```python
from build123d import *

# Parameters (mm, degrees)
F0_W     = 50
F0_H     = 80
F1_DEPTH = 60
F3_DEPTH = 80.001
F6_DEPTH = 66.156149
F7_W     = 5
F7_H     = 12.45938
F8_DEPTH = 43.57978


with BuildPart() as f1:
    # F0 (on Top) → F1 (new body)
    with BuildSketch(Plane.XY):
        with Locations((25, 40)):
            Rectangle(F0_W, F0_H)
    extrude(amount=F1_DEPTH)

    # F2 (on face) → F3 (cut, through all)
    with BuildSketch(Plane.XZ):
        Polygon((50, 20.009331), (50, 60), (15.790775, 60), align=None)
    extrude(amount=-F3_DEPTH, mode=Mode.SUBTRACT)

    # F5 (on offset) → F6 (cut)
    with BuildSketch(Plane.YZ.offset(50)):
        Polygon((0, 65.009331), (0, 20.009331), (36.240832, 65.009331), align=None)
    extrude(amount=-F6_DEPTH, mode=Mode.SUBTRACT)

    # F7 (on face) → F8 (cut)
    with BuildSketch(Plane(origin=(0, 0, 0), x_dir=(0, -1, 0), z_dir=(-1, 0, 0))):
        with Locations((-53.603279, 53.77031)):
            Rectangle(F7_W, F7_H)
        with Locations((-58.603279, 53.77031)):
            Rectangle(F7_W, F7_H)
    extrude(amount=-F8_DEPTH, mode=Mode.SUBTRACT)


solid = f1.part
```
Could you check a few things on this model? Use its own coordinates, in mm. A direction names the side the tool comes from. Round coordinates to 2 decimals unless told otherwise and drop trailing zeros. Write each loop counter-clockwise with the first axis right and the second up, starting at its lowest first coordinate (ties: lowest second). Pieces come first, ordered by that corner, then holes.
(1) Thinking about a two-plate mould opening in Y: for faces 1 (the face through (13, 56, 47.541)), 2 (the face through (8, 71, 60)), 3 (the face through (25, 0, 10)), which applies, +Y half, -Y half, draft (parallel to the pull), parting line (faces both ways), or undercut?
Findings below:
face 1: undercut
face 2: draft
face 3: -Y half
(2) Suppose I cut it at D-D on z = 44. Write out the boundary of the cut face in (x, y).
Findings below:
outline: (0, 19.32) - (29.48, 19.32) - (29.48, 80) - (0, 80) - close
(3) Suppose I cut it at B-B on z = 52. Write out the boundary of the cut face in (x, y).
Findings below:
outline: (0, 25.76) - (22.63, 25.76) - (22.63, 51.1) - (0, 51.1) - close; (0, 61.1) - (22.63, 61.1) - (22.63, 80) - (0, 80) - close
(4) Suppose I cut it at C-C on y = 39. Write out the boundary of the cut face in (x, z), and give its area (3 significant figures).
Findings below:
outline: (0, 0) - (50, 0) - (50, 20.01) - (15.79, 60) - (0, 60) - close
area: 2,320 mm2
(5) Suppose I cut it at A-A on x = 12.5. Write out the boundary of the cut face in (y, z), and give its area (3 significant figures).
Findings below:
outline: (0, 0) - (80, 0) - (80, 60) - (61.1, 60) - (61.1, 47.54) - (51.1, 47.54) - (51.1, 60) - (32.21, 60) - (0, 20.01) - close
area: 4,030 mm2
(6) Which directions (+Z, -Z, +X, -X, +Y, -Y) give clear straight access to the entire face, cutting with the end or side of a thin tool? Please do faces 4 (the face through (10, 51.103, 54)), 5 (the face through (19, 80, 23)).
Findings below:
face 4: +Z, +X, -X
face 5: +Z, -Z, +X, -X, +Y
(7) If I drill on probe 1 along Y at (x, z) = (13, 52); probe 2 along X at (y, z) = (47.5, 48); probe 3 along Z at (x, y) = (20, 62), over which ranges is the centre line in solid material (lowest first)?
Findings below:
probe 1: y = 25.76 to 51.1, 61.1 to 80
probe 2: x = 0 to 26.06
probe 3: z = 0 to 55.08
(8) For pin 1 (1 mm diameter, centred on x = 30.5, z = 28.5, fed in from -Y); pin 2 (5 mm diameter, centred on x = 18.5, y = 56.5, fed in from +Z); pin 3 (8 mm diameter, centred on x = 5.5, z = 36.5, fed in from -Y), each with a flat end and sliding along its axis, tell me the tip position at first contact or that it passes through.
Findings below:
pin 1: stops at y = 6.44
pin 2: stops at z = 47.54
pin 3: stops at y = 10.06
